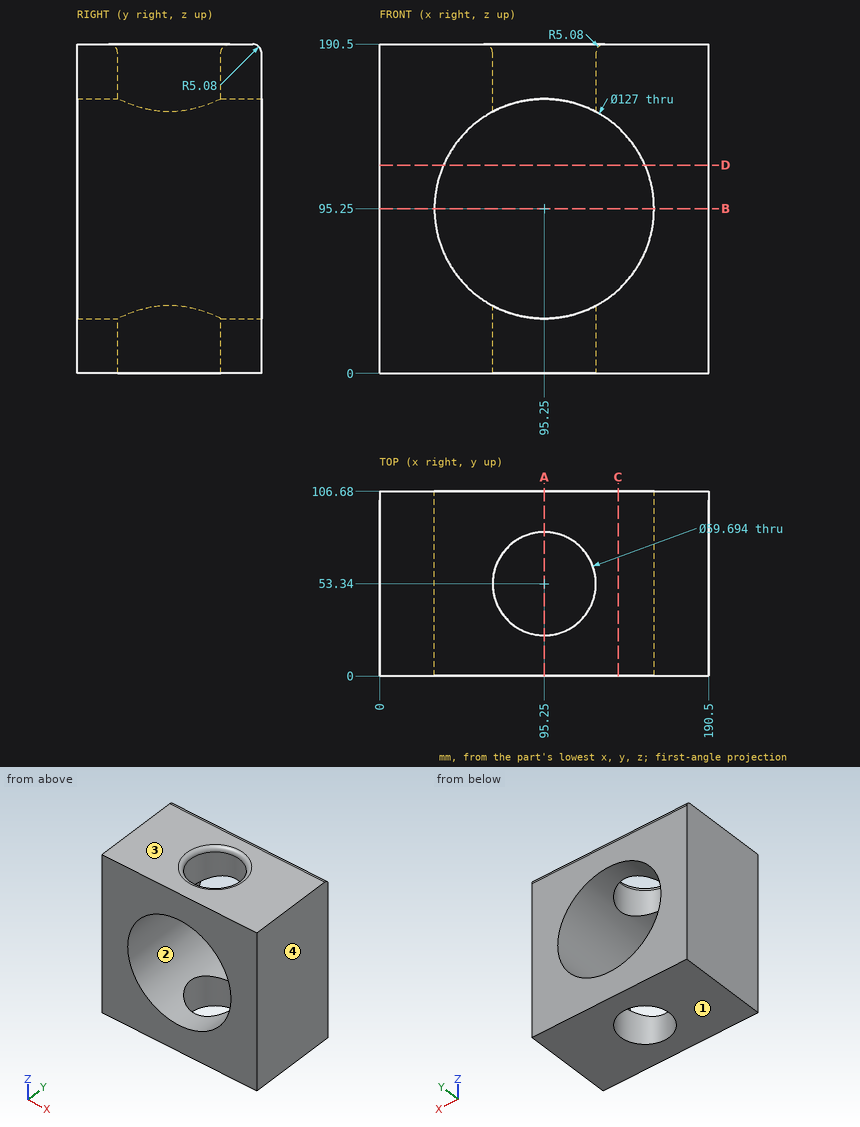
Source: three-view drawing plus pictorial views. Frame: mm from the lowest corner of the part. Give positions to 0.01 mm unless a question says otherwise; leave off trailing zeros. Order: outer loops, then holes, each group sorted by start corner. A loop starts at its lowest first (then second) coordinate and runs counter-clockwise, first axis right, second up. Notation, with made-up numbers: (84, -36.5) - (131, -36.5) arc R20 cw to (131, -20.5) - close; hole circle Ø4 at (83, 79). An arc over 180 degrees is marked (long way). Answer as a JSON object with one key per item and string values. Group by question number.
Q1. Line query: probe 1 along Y at (x, z) = (94, 170); probe 2 along X at (y, z) = (53, 13) (1 decimal); probe 3 along X at (y, z) = (70.5, 166). Output: solid intervals per line, ascending.
Q2. Cut plane A-A, the plane x = 95.25. Output: boundary loops of the cut face in (y, z).
Q3. Cut plane C-C, the plane x = 138. Output: boundary loops of the cut face in (y, z), then the cut area to 3 significant figures.
Q4. Cut plane D-D, the plane z = 120.5. Output: boundary loops of the cut face in (x, y).
Q5. Mould query, pull axis Z, two halves, no side actions, for the marked faces 1, 2, 3 and 4. Classes: pulls with the +Z half, pulls with the -Z half, needs draft (parallel to the pull), parting line crosses it, or undercut.
Q6. Cut plane B-B, the plane z = 95.25. Output: boundary loops of the cut face in (x, y).
Results:
{
 "1": {"probe 1": "0 to 23.52, 83.16 to 106.68", "probe 2": "0 to 65.4, 125.1 to 190.5", "probe 3": "0 to 70.83, 119.67 to 190.5"},
 "2": {"outline": "(0, 0) - (23.49, 0) - (23.49, 31.75) - (0, 31.75) - close; (0, 158.75) - (23.49, 158.75) - (23.49, 185.42) arc R5.08 ccw to (18.41, 190.5) - (0, 190.5) - close; (83.19, 0) - (106.68, 0) - (106.68, 31.75) - (83.19, 31.75) - close; (83.19, 158.75) - (106.68, 158.75) - (106.68, 185.42) arc R5.08 ccw to (101.6, 190.5) - (88.27, 190.5) arc R5.08 ccw to (83.19, 185.42) - close"},
 "3": {"outline": "(0, 0) - (106.68, 0) - (106.68, 48.3) - (0, 48.3) - close; (0, 142.2) - (106.68, 142.2) - (106.68, 185.42) arc R5.08 ccw to (101.6, 190.5) - (0, 190.5) - close", "area": "10,300 mm^2"},
 "4": {"outline": "(0, 0) - (36.99, 0) - (36.99, 106.68) - (0, 106.68) - close; (153.51, 0) - (190.5, 0) - (190.5, 106.68) - (153.51, 106.68) - close"},
 "5": {"face 1": "pulls with the -Z half", "face 2": "undercut", "face 3": "pulls with the +Z half", "face 4": "needs draft"},
 "6": {"outline": "(0, 0) - (31.75, 0) - (31.75, 106.68) - (0, 106.68) - close; (158.75, 0) - (190.5, 0) - (190.5, 106.68) - (158.75, 106.68) - close"}
}
